Geometry check sheet. Reference: the model listing, model coordinates, mm. A direction names the side the tool comes from. Round coordinates to 2 decimals unless told otherwise and drop trailing zeros. Write each loop counter-clockwise with the first axis right and the second up, starting at its lowest first coordinate (ties: lowest second). Pieces come first, ordered by that corner, then holes.
Item 1: Access from +Z, -Z, +X, -X, +Y, -Y to the whole of each face (thin tool, end or side, straight path). Record for faces 4 (the face through (-6, 0, 7)), 5 (the face through (-64.8, -11, -37.3)).
Item 2: Scan lines: probe 1 along X at (y, z) = (-14.5, -20); probe 2 along Z at (x, y) = (-47, -16.5); probe 3 along Z at (x, y) = (-38.5, -3.75). Record each from-to range of solid material in increasing order.
Item 3: Cross-section at D-D (x = 12.5). Enter the section's corners in (y, z) (3 decimals), then the cut area to 3 significant figures.
Item 4: Cross-section at B-B (z = 22). Enter the section's corners in (x, y) (3 decimals), then the cut area to 3 significant figures.
Item 5: Depth check by flat-ended pin: P1, Ø1, axis at x = 41, z = 29, coming from the +Y side; P2, Ø6, axis at x = -22.5, z = -14, coming from the -Y side (3 decimals). Enter the tip coordinate at first touch or a pass-through.
Item 6: Cross-section at C-C (x = -32). Enter the section's corners in (y, z) (3 decimals).
Item 7: Cross-section at A-A (y = -9.75). Enter the section's corners in (x, z) (3 decimals), then the cut area to 3 significant figures.
Item 8: Draft check along Z on faces 1 (the face through (15, -6.35, 10)), 2 (the face through (-71.788, -9, 6)), 3 (the face through (-6, -9, -44.105)). Enter one of: pulls with the +Z half, pulls with the -Z half, needs draft (parallel to the pull), parting line crosses it, or undercut.
from build123d import *

# Parameters (mm, degrees)
F0_W     = 133.35
F0_H     = 101.6
F1_DEPTH = 19.05
F2_T     = -3.175
F3_R     = 6.35
F4_DEPTH = 3.175
F5_R     = 3.175
F6_DEPTH = 12.7
F7_R     = 3.175
F8_DEPTH = 12.7
F9_R     = 12.7
F10_SIZE = 1.6002


with BuildPart() as f1:
    # F0 (on Front) → F1 (new body)
    with BuildSketch(Plane.XZ):
        with Locations((-5.1130652428, 6.6948301531)):
            Rectangle(F0_W, F0_H)
    extrude(amount=F1_DEPTH)

    # F2
    f2_openings = [f1.faces().sort_by_distance(p)[0] for p in [
        (-5.113065, -19.05, 6.69483),
    ]]
    offset(amount=F2_T, openings=f2_openings)

    # F3 (on face) → F4 (join)
    with BuildSketch(Plane.XZ.offset(3.175)):
        with Locations((-43.2130652428, 6.6948301531)):
            Circle(F3_R)
        with Locations((13.9369347572, 6.6948301531)):
            Circle(F3_R)
    extrude(amount=F4_DEPTH)

    # F5 (on face) → F6 (join)
    with BuildSketch(Plane.XZ.offset(6.35)):
        with Locations((-43.2130652428, 6.6948301531)):
            Circle(F5_R)
    extrude(amount=F6_DEPTH)

    # F7 (on face) → F8 (join)
    with BuildSketch(Plane.XZ.offset(6.35)):
        with Locations((13.9369347572, 6.6948301531)):
            Circle(F7_R)
    extrude(amount=F8_DEPTH)

    # F9
    f9_edges = [f1.edges().sort_by_distance(p)[0] for p in [
        (-68.613065, -11.1125, -40.93017),
        (58.386935, -11.1125, -40.93017),
        (-68.613065, -11.1125, 54.31983),
        (58.386935, -11.1125, 54.31983),
    ]]
    fillet(f9_edges, radius=F9_R)

    # F10
    f10_edges = [f1.edges().sort_by_distance(p)[0] for p in [
        (61.561935, -19.05, 6.69483),
        (-5.113065, -19.05, -44.10517),
        (-71.788065, -19.05, 6.69483),
        (-5.113065, -19.05, 57.49483),
    ]]
    chamfer(f10_edges, length=F10_SIZE)


solid = f1.part
Resolved:
1. face 4: +Z, -Z, +X, -X, +Y
1. face 5: -Y
2. probe 1: x = -71.79 to -68.61, 58.39 to 61.56
2. probe 2: z = -44.11 to -40.93, 54.32 to 57.49
2. probe 3: z = -44.11 to -40.93, 2.44 to 10.95, 54.32 to 57.49
3. outline: (-19.05, -42.505) - (-17.45, -44.105) - (0, -44.105) - (0, 57.495) - (-17.45, 57.495) - (-19.05, 55.895) - (-19.05, 54.32) - (-3.175, 54.32) - (-3.175, 12.88) - (-6.35, 12.88) - (-6.35, 9.526) - (-19.05, 9.526) - (-19.05, 3.864) - (-6.35, 3.864) - (-6.35, 0.51) - (-3.175, 0.51) - (-3.175, -40.93) - (-19.05, -40.93) - close
3. area: 532 mm2
4. outline: (-71.788, -17.45) - (-70.188, -19.05) - (-68.613, -19.05) - (-68.613, -3.175) - (58.387, -3.175) - (58.387, -19.05) - (59.962, -19.05) - (61.562, -17.45) - (61.562, 0) - (-71.788, 0) - close
4. area: 522 mm2
5. P1: stops at y = 0
5. P2: stops at y = -3.175
6. outline: (-19.05, -42.505) - (-17.45, -44.105) - (0, -44.105) - (0, 57.495) - (-17.45, 57.495) - (-19.05, 55.895) - (-19.05, 54.32) - (-3.175, 54.32) - (-3.175, -40.93) - (-19.05, -40.93) - close
7. outline: (-71.788, -44.105) - (61.562, -44.105) - (61.562, 57.495) - (-71.788, 57.495) - close; circle Ø6.35 at (-43.213, 6.695); circle Ø6.35 at (13.937, 6.695); hole (-68.613, -28.23) arc R12.7 ccw to (-55.913, -40.93) - (45.687, -40.93) arc R12.7 ccw to (58.387, -28.23) - (58.387, 41.62) arc R12.7 ccw to (45.687, 54.32) - (-55.913, 54.32) arc R12.7 ccw to (-68.613, 41.62) - close
7. area: 1,650 mm2
8. face 1: undercut
8. face 2: needs draft
8. face 3: pulls with the -Z half
